from build123d import *

# Parameters (mm, degrees)
SKETCH1_W           = 50.8
SKETCH1_H           = 50.8
BOSS_EXTRUDE1_DEPTH = 48.26
SKETCH2_W           = 45.72
SKETCH2_H           = 45.72
CUT_EXTRUDE1_DEPTH  = 45.72
SKETCH3_W           = 48.26
SKETCH3_H           = 48.26
CUT_EXTRUDE2_DEPTH  = 2.54


with BuildPart() as part:
    # Sketch1 → Boss-Extrude1 (new body)
    with BuildSketch(Plane(origin=(0, 0, 0), x_dir=(1, 0, 0), z_dir=(0, 1, 0))):
        with Locations((25.4, 25.4)):
            Rectangle(SKETCH1_W, SKETCH1_H)
    extrude(amount=BOSS_EXTRUDE1_DEPTH)

    # Sketch2 → Cut-Extrude1 (cut)
    with BuildSketch(Plane(origin=(0, 48.26, 0), x_dir=(1, 0, 0), z_dir=(0, 1, 0))):
        with Locations((25.4, 25.4)):
            Rectangle(SKETCH2_W, SKETCH2_H)
    extrude(amount=-CUT_EXTRUDE1_DEPTH, mode=Mode.SUBTRACT)

    # Sketch3 → Cut-Extrude2 (cut)
    with BuildSketch(Plane(origin=(0, 48.26, 0), x_dir=(1, 0, 0), z_dir=(0, 1, 0))):
        with Locations((25.4, 25.4)):
            Rectangle(SKETCH3_W, SKETCH3_H)
    extrude(amount=-CUT_EXTRUDE2_DEPTH, mode=Mode.SUBTRACT)


solid = part.part
For this review, take the finished solid that the model builds, in its own axes (mm). A direction names the side the tool comes from. Round coordinates to 2 decimals unless told otherwise and drop trailing zeros. Write each loop counter-clockwise with the first axis right and the second up, starting at its lowest first coordinate (ties: lowest second). Pieces come first, ordered by that corner, then holes. Notation, with made-up numbers: M 85.25,22 L 105.25,22 A14 cw 105.25,36 Z; hole C -35,62.5 d5. An arc over 180 degrees is marked long. Write item = value, one per line. Start each with the question number.
(1) For faces 4 (the face through (48.26, 24, -25)), 5 (the face through (25, 24, -50.8)), list the 3-axis set-ups (+Z, -Z, +X, -X, +Y, -Y) from which the entire face can be reached by the end or side of a thin tool; tool diameter is ignored.
(2) For line 1 along X through (y, z) = (19, -37.5); line 2 along Z through (x, y) = (35.5, 28.5); line 3 along Y through (x, z) = (9, -40.5), list the stretches that pass through material, from the lowest coordinate up.
(3) We need section B-B (z = -12.5). Give the boundary of the cut face in (x, y), then the cut area to 3 significant figures.
(4) Clearance check with a flat-ended pin moving along its axis: pin 1 Ø1 at (x, z) = (40, -6) entering from +Y. State where the tip first meets the part, or that it passes through.
(5) The part is to be moulded in two halves that separate along Z. For faces 1 (the face through (25, 47, -1.27)), 2 (the face through (23, 48.26, -1)), 3 (the face through (25, 24, 0)), say which applies: +Z half, -Z half, draft (parallel to the pull), parting line (faces both ways), or undercut.
(6) We need section A-A (y = 22.5). Give the boundary of the cut face in (x, z).
(7) We need section C-C (x = 14.5). Give the boundary of the cut face in (y, z).
Results found:
q1.face_4 = +Y
q1.face_5 = -Z, +X, -X, +Y, -Y
q2.line_1 = 0 to 2.54, 48.26 to 50.8
q2.line_2 = -50.8 to -48.26, -2.54 to 0
q2.line_3 = 0 to 2.54
q3.outline = M 0,0 L 50.8,0 L 50.8,48.26 L 49.53,48.26 L 49.53,45.72 L 48.26,45.72 L 48.26,2.54 L 2.54,2.54 L 2.54,45.72 L 1.27,45.72 L 1.27,48.26 L 0,48.26 Z
q3.area = 355 mm²
q4.pin_1 = 2.54
q5.face_1 = undercut
q5.face_2 = draft
q5.face_3 = +Z half
q6.outline = M 0,-50.8 L 50.8,-50.8 L 50.8,0 L 0,0 Z; hole M 2.54,-48.26 L 48.26,-48.26 L 48.26,-2.54 L 2.54,-2.54 Z
q7.outline = M 0,-50.8 L 48.26,-50.8 L 48.26,-49.53 L 45.72,-49.53 L 45.72,-48.26 L 2.54,-48.26 L 2.54,-2.54 L 45.72,-2.54 L 45.72,-1.27 L 48.26,-1.27 L 48.26,0 L 0,0 Z
